Source: CAD feature listing. Evaluate the final solid. Frame: model axes, mm. Face numbers are marked on the shaded views. Give positions to 0.01 mm unless a question says otherwise; leave off trailing zeros. Write each loop counter-clockwise with the first axis right and the second up, starting at its lowest first coordinate (ties: lowest second). Pieces come first, ordered by that corner, then holes. Notation, with made-up numbers: (56, -27.75) -> (86, -27.75) arc R26 ccw to (86, -2.75) -> close; hole circle Ø6 at (-13.75, 46.5). An arc over 180 degrees is marked (long way). Answer as a JSON object with one key per item and string values. Group by question number.
Item 1: Section query D-D on z = 13. Give the number of separate pieces and of enclosed holes in the cut face, plus the area to 3 significant figures.
Item 2: Section query B-B on x = 50.8. Return the cut outline in (y, z) (3 decimals).
Item 3: First-contact query: pin 1 Ø14.5 at (x, y) = (50.8, -68.25) entering from +Z (3 decimals); pin 2 Ø7 at (x, y) = (50.8, 68.25) entering from +Z. Flat tips, straight axial feed; report the tip coordinate or a pass-through.
Item 4: Section query A-A on y = 0. Return the cut outline in (x, z) (3 decimals), plus the area to 3 significant figures.
Item 5: Section query C-C on x = 0. Return the cut outline in (y, z) (3 decimals).
Item 6: Pull-direction query (Y, two-part tool) for the marked faces 1, 2, 3 and 4; classes: pulls with the +Y half, pulls with the -Y half, needs draft (parallel to the pull), parting line crosses it, or undercut.
Item 7: Ray query, probe 1 along Y at (x, z) = (50.8, 7.25); probe 2 along X at (y, z) = (32.5, 1.25); probe 3 along X at (y, z) = (-1, 4). Return the intervals inside material, ascending. Write a range as from..to.
from build123d import *

# Parameters (mm, degrees)
F0_W     = 102.87
F0_H     = 152.4
F0_R     = 4.5212
F1_DEPTH = 15.875
F2_DEPTH = 197
F3_R     = 36.4998
F4_DEPTH = 15.876
F5_R     = 4.5212
F6_DEPTH = 15.876


# Not quite as in the source:
# - an extrude ends at something that could not be found from the text; its depth is read off the source's solid


with BuildPart() as f1:
    # F0 (on Top) → F1 (new body)
    with BuildSketch(Plane.XY):
        with Locations((8.763, 0)):
            Rectangle(F0_W, F0_H)
        with Locations((-31.75, -68.2498)):
            Circle(F0_R, mode=Mode.SUBTRACT)
        with Locations((50.8, -68.2498)):
            Circle(F0_R, mode=Mode.SUBTRACT)
        with Locations((-31.75, 68.2498)):
            Circle(F0_R, mode=Mode.SUBTRACT)
        with Locations((50.8, 68.2498)):
            Circle(F0_R, mode=Mode.SUBTRACT)
    extrude(amount=F1_DEPTH)

    # F0 (on Top) → F2 (cut, through all)
    with BuildSketch(Plane.XY):
        with Locations((8.763, 0)):
            Rectangle(F0_W, F0_H)
        with Locations((-31.75, -68.2498)):
            Circle(F0_R, mode=Mode.SUBTRACT)
        with Locations((50.8, -68.2498)):
            Circle(F0_R, mode=Mode.SUBTRACT)
        with Locations((-31.75, 68.2498)):
            Circle(F0_R, mode=Mode.SUBTRACT)
        with Locations((50.8, 68.2498)):
            Circle(F0_R, mode=Mode.SUBTRACT)
    extrude(amount=-F2_DEPTH, mode=Mode.SUBTRACT)

    # F3 (on face) → F4 (cut, through all)
    with BuildSketch(Plane.XY.offset(15.875)):
        Circle(F3_R)
    extrude(amount=-F4_DEPTH, mode=Mode.SUBTRACT)

    # F5 (on face) → F6 (cut, through all)
    with BuildSketch(Plane.XY.offset(15.875)):
        with Locations((-34.6456, 34.6456)):
            Circle(F5_R)
        with Locations((34.6456, 34.6456)):
            Circle(F5_R)
        with Locations((34.6456, -34.6456)):
            Circle(F5_R)
        with Locations((-34.6456, -34.6456)):
            Circle(F5_R)
    extrude(amount=-F6_DEPTH, mode=Mode.SUBTRACT)


solid = f1.part
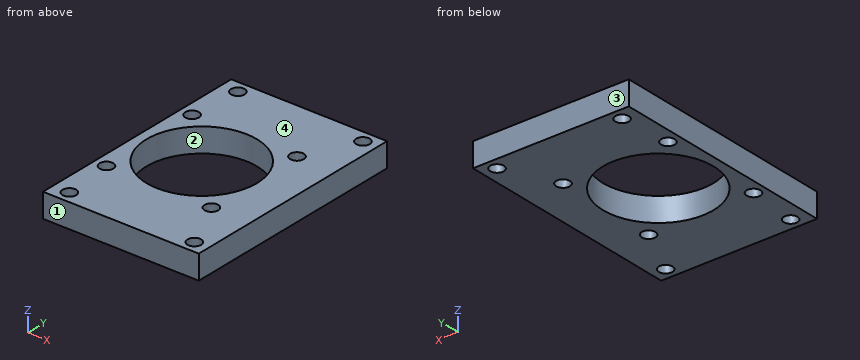
Worked answers:
{
 "1": {"separate pieces": "1", "enclosed holes": "9", "area": "11,000 mm^2"},
 "2": {"outline": "(-76.2, 0) -> (-72.771, 0) -> (-72.771, 15.875) -> (-76.2, 15.875) -> close; (-63.729, 0) -> (63.729, 0) -> (63.729, 15.875) -> (-63.729, 15.875) -> close; (72.771, 0) -> (76.2, 0) -> (76.2, 15.875) -> (72.771, 15.875) -> close"},
 "3": {"pin 1": "z = 15.875", "pin 2": "through"},
 "4": {"outline": "(-42.672, 0) -> (-36.5, 0) -> (-36.5, 15.875) -> (-42.672, 15.875) -> close; (36.5, 0) -> (60.198, 0) -> (60.198, 15.875) -> (36.5, 15.875) -> close", "area": "474 mm^2"},
 "5": {"outline": "(-76.2, 0) -> (-36.5, 0) -> (-36.5, 15.875) -> (-76.2, 15.875) -> close; (36.5, 0) -> (76.2, 0) -> (76.2, 15.875) -> (36.5, 15.875) -> close"},
 "6": {"face 1": "pulls with the -Y half", "face 2": "undercut", "face 3": "pulls with the +Y half", "face 4": "needs draft"},
 "7": {"probe 1": "-76.2..-72.77, -63.73..63.73, 72.77..76.2", "probe 2": "-42.67..-38.63, -30.67..-16.61, 16.61..30.67, 38.63..60.2", "probe 3": "-42.67..-36.49, 36.49..60.2"}
}
